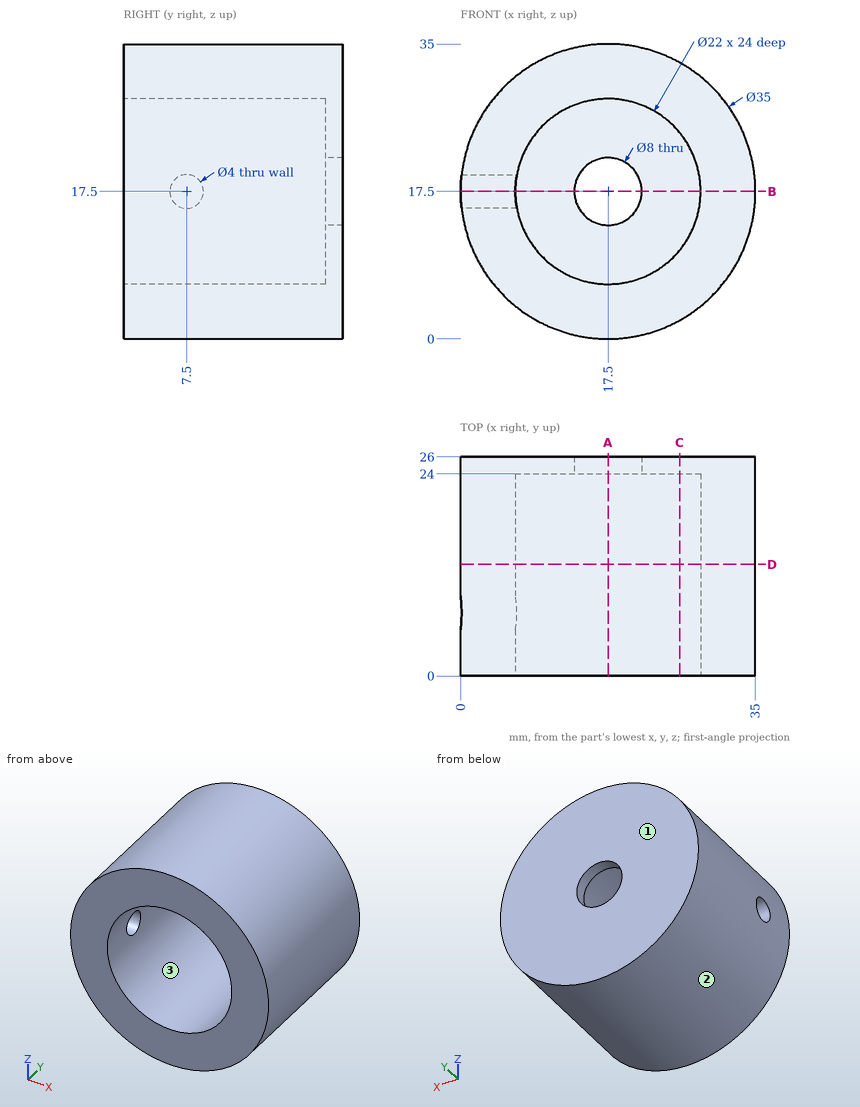
Could you check a few things on this drawing? It's one solid part, dimensions in mm from its lowest x, y, z. Round coordinates to 2 decimals unless told otherwise and drop trailing zeros. Order: outer loops, then holes, each group sorted by start corner. A loop starts at its lowest first (then second) coordinate and runs counter-clockwise, first axis right, second up. Notation, with made-up numbers: (44.25, 31.25) -> (64.25, 31.25) arc R19 ccw to (64.25, 52.25) -> close; hole circle Ø7 at (33, 75.25). An arc over 180 degrees is marked (long way). One line per question, with ' | ' between items.
Q1. If we section it at A-A on x = 17.5: Write out the boundary of the cut face in (y, z), plus the area to 3 significant figures.
Computed values:
outline: (0, 0) -> (26, 0) -> (26, 13.5) -> (24, 13.5) -> (24, 6.5) -> (0, 6.5) -> close; (0, 28.5) -> (24, 28.5) -> (24, 21.5) -> (26, 21.5) -> (26, 35) -> (0, 35) -> close | area: 366 mm²
Q2. We'd pull the mould along X, two halves only. Please class the marked faces 1, 2 and 3: released by +X, released by -X, zero draft, split by the parting line, or undercut.
Computed values:
face 1: zero draft | face 2: split by the parting line | face 3: undercut
Q3. I'm going to push flat-ended pins straight in: pin 1 (10 mm diameter, centred on y = 3, z = 8.5, fed in from -X); pin 2 (12 mm diameter, centred on x = 21.5, z = 16.5, fed in from -Y); pin 3 (4 mm diameter, centred on x = 24, y = 11, fed in from +Z). Where does each tip first touch, or does it pass through?
Computed values:
pin 1: x = 0.46 | pin 2: y = 24 | pin 3: z = 34.41
Q4. If I drill on line 1 (Z direction, x = 17.5, y = 7.5); line 2 (Z direction, x = 17.5, y = 24.95); line 3 (Y direction, x = 21, z = 22), over which ranges is the centre line in solid material (lowest first)? Write a range as from..to.
Computed values:
line 1: 0..6.5, 28.5..35 | line 2: 0..13.5, 21.5..35 | line 3: 24..26
Q5. If we section it at B-B on z = 17.5: Write out the boundary of the cut face in (x, y).
Computed values:
outline: (0, 0) -> (6.5, 0) -> (6.5, 5.5) -> (0, 5.5) -> close; (0, 9.5) -> (6.5, 9.5) -> (6.5, 24) -> (13.5, 24) -> (13.5, 26) -> (0, 26) -> close; (21.5, 24) -> (28.5, 24) -> (28.5, 0) -> (35, 0) -> (35, 26) -> (21.5, 26) -> close
Q6. If we section it at D-D on y = 13.25: Write out the boundary of the cut face in (x, z), plus the area to 3 significant figures.
Computed values:
outline: circle Ø35 at (17.5, 17.5); hole circle Ø22 at (17.5, 17.5) | area: 582 mm²
Q7. If we section it at C-C on x = 26: Write out the boundary of the cut face in (y, z), plus the area to 3 significant figures.
Computed values:
outline: (0, 2.2) -> (26, 2.2) -> (26, 32.8) -> (0, 32.8) -> (0, 24.48) -> (24, 24.48) -> (24, 10.52) -> (0, 10.52) -> close | area: 460 mm²
